```python
from build123d import *

# Parameters (mm, degrees)
SOCKETRIGHT_R                       = 16.7005
SOCKETRIGHT_DEPTH                   = 31.4325
SOCKETRIGHT_PITCH_ANGLE             = 90
SOCKETTOP_R                         = 16.7005
SOCKETTOP_DEPTH                     = 31.4325
SOCKETBOTTOM_R                      = 16.7005
SOCKETBOTTOM_DEPTH                  = 31.4325
SOCKETLEFT_R                        = 16.7005
SOCKETLEFT_DEPTH                    = 31.4325
SOCKETLEFT_PITCH_ANGLE              = 90
OBJ1_R           = 13.0683
OBJ1_DEPTH       = 108.2675
OBJ1_PITCH_ANGLE = 90
OBJ2             = 13.0683
OBJ3         = 108.2675
OBJ4_R           = 20.6375
OBJ4_DEPTH       = 98.425
OBJ4_PITCH_ANGLE = 90
OBJ5             = 20.6375
OBJ6         = 98.425


with BuildPart() as socketright:
    # SocketRight → SocketRight (new body)
    with BuildSketch(Plane.XY):
        Circle(SOCKETRIGHT_R)
    extrude(amount=SOCKETRIGHT_DEPTH)


with BuildPart() as socketright_1:
    # SocketRight pitch: moved
    add(socketright.part.rotate(Axis((0, 0, 0), (0, 1, 0)), SOCKETRIGHT_PITCH_ANGLE))


with BuildPart() as socketright_2:
    # SocketRight placement: moved
    add(socketright_1.part.moved(Location((20.6375, 0, 0))))


with BuildPart() as sockettop:
    # SocketTop → SocketTop (new body)
    with BuildSketch(Plane.XY.offset(20.6375)):
        Circle(SOCKETTOP_R)
    extrude(amount=SOCKETTOP_DEPTH)


with BuildPart() as socketbottom:
    # SocketBottom → SocketBottom (new body)
    with BuildSketch(Plane.XY.offset(-52.07)):
        Circle(SOCKETBOTTOM_R)
    extrude(amount=SOCKETBOTTOM_DEPTH)


with BuildPart() as sockets:
    # SocketLeft → SocketLeft (new body)
    with BuildSketch(Plane.XY):
        Circle(SOCKETLEFT_R)
    extrude(amount=SOCKETLEFT_DEPTH)


with BuildPart() as sockets_1:
    # SocketLeft pitch: moved
    add(sockets.part.rotate(Axis((0, 0, 0), (0, 1, 0)), SOCKETLEFT_PITCH_ANGLE))


with BuildPart() as sockets_2:
    # SocketLeft placement: moved
    add(sockets_1.part.moved(Location((-52.07, 0, 0))))

    # Sockets: union SocketRight, SocketTop, SocketBottom
    add(socketright_2.part)
    add(sockettop.part)
    add(socketbottom.part)


with BuildPart() as obj1:
    # obj1 → obj1 (new body)
    with BuildSketch(Plane.XY):
        Circle(OBJ1_R)
    extrude(amount=OBJ1_DEPTH)


with BuildPart() as obj1_1:
    # obj1 pitch: moved
    add(obj1.part.rotate(Axis((0, 0, 0), (0, 1, 0)), OBJ1_PITCH_ANGLE))


with BuildPart() as obj1_2:
    # obj1 placement: moved
    add(obj1_1.part.moved(Location((-54.13375, 0, 0))))


with BuildPart() as innercrossfusion:
    with BuildSketch(Plane.XY.offset(-54.13375)):
        Circle(OBJ2)
    extrude(amount=OBJ3)

    # InnerCrossFusion: union obj1
    add(obj1_2.part)


with BuildPart() as obj4:
    # obj4 → obj4 (new body)
    with BuildSketch(Plane.XY):
        Circle(OBJ4_R)
    extrude(amount=OBJ4_DEPTH)


with BuildPart() as obj4_1:
    # obj4 pitch: moved
    add(obj4.part.rotate(Axis((0, 0, 0), (0, 1, 0)), OBJ4_PITCH_ANGLE))


with BuildPart() as obj4_2:
    # obj4 placement: moved
    add(obj4_1.part.moved(Location((-49.2125, 0, 0))))


with BuildPart() as cross:
    with BuildSketch(Plane.XY.offset(-49.2125)):
        Circle(OBJ5)
    extrude(amount=OBJ6)

    # OuterCrossFusion: union obj4
    add(obj4_2.part)

    # Cut: cut InnerCrossFusion
    add(innercrossfusion.part, mode=Mode.SUBTRACT)

    # Cross: cut Sockets
    add(sockets_2.part, mode=Mode.SUBTRACT)


solid = cross.part
```
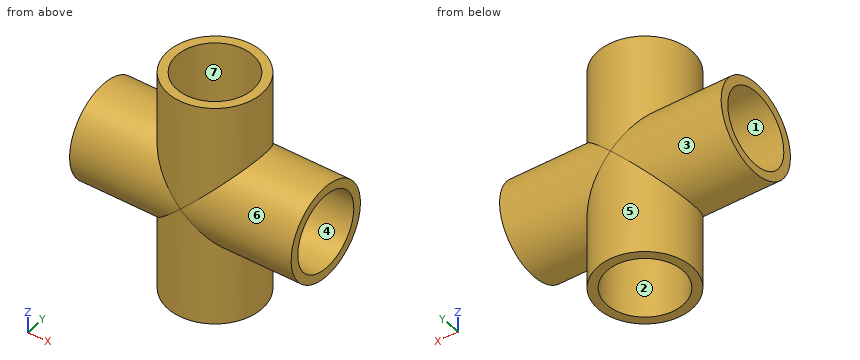
Geometry check sheet. Reference: the model listing, model coordinates, mm. Face numbers are marked on the shaded views. A direction names the side the tool comes from. Round coordinates to 2 decimals unless told otherwise and drop trailing zeros. Order: outer loops, then holes, each group sorted by start corner. A loop starts at its lowest first (then second) coordinate and runs counter-clockwise, first axis right, second up. Notation, with made-up numbers: (-2.75, 75.5) - (5.25, 75.5) arc R13 ccw to (5.25, 82.5) - close; hole circle Ø3 at (58.25, -10.75). An arc over 180 degrees is marked (long way). Use a Markdown table: item, result. Add a question column.
1) Section check A-A (z = 11.5). Record the cut outline in (x, y) (1 decimal), then the cut area to 3 significant figures.
2) Thickness scan on line 1 along Y through (x, z) = (-30.5, 0). Record the ranges inside material, lowest first.
3) Section check B-B (x = -15). Record the cut outline in (y, z) (1 decimal), then the cut area to 3 significant figures.
4) Section check D-D (z = -15). Record the cut outline in (x, y) (1 decimal).
5) Gauge pin test, flat ends, axial feed: P1, Ø20, axis at x = 0, y = 0, coming from the +Z side; P2, Ø12, axis at x = 1.5, z = -32, coming from the +Y side; P3, Ø16.5, axis at x = -3, y = -4.5, coming from the -Z side; P4, Ø6, axis at y = -15.5, z = -23.5, coming from the +X side. Record the tip position at first contact, or that the pin passes through.
6) Set-up check for the marked faces 5, 6 and 7: record each of +Z, -Z, +X, -X, +Y, -Y from which the full face is reachable in a straight line by a thin tool's end or side.
7) Mould release check, pull along Z, two halves, no side actions. Record for the marked faces 1, 2, 3 and 4: released by +Z, released by -Z, zero draft, split by the parting line, or undercut.
8) Section check C-C (y = 0). Count the separate pieces of the cut face and the enclosed holes in it, then the cut area to 3 significant figures.
Established:
| question | item | result |
|---|---|---|
| 1 | outline | (-49.2, -17.1) - (-11.5, -17.1) arc R20.6 ccw to (11.5, -17.1) - (49.2, -17.1) - (49.2, -12.1) - (20.6, -12.1) - (20.6, -6.2) - (11.5, -6.2) arc R13.1 cw to (-11.5, -6.2) - (-20.6, -6.2) - (-20.6, -12.1) - (-49.2, -12.1) - close; (-49.2, 12.1) - (-20.6, 12.1) - (-20.6, 6.2) - (-11.5, 6.2) arc R13.1 cw to (11.5, 6.2) - (20.6, 6.2) - (20.6, 12.1) - (49.2, 12.1) - (49.2, 17.1) - (11.5, 17.1) arc R20.6 ccw to (-11.5, 17.1) - (-49.2, 17.1) - close |
| 1 | area | 1,360 mm2 |
| 2 | line 1 | -20.64 to -16.7, 16.7 to 20.64 |
| 3 | outline | (-14.2, -49.2) - (-7.3, -49.2) - (-7.3, -20.6) - (7.3, -20.6) - (7.3, -49.2) - (14.2, -49.2) - (14.2, -15) arc R20.6 ccw to (14.2, 15) - (14.2, 49.2) - (7.3, 49.2) - (7.3, 20.6) - (-7.3, 20.6) - (-7.3, 49.2) - (-14.2, 49.2) - (-14.2, 15) arc R20.6 ccw to (-14.2, -15) - close; hole circle Ø26.1 at (0, 0) |
| 3 | area | 1,680 mm2 |
| 4 | outline | (-49.2, -14.2) - (-15, -14.2) arc R20.6 ccw to (15, -14.2) - (49.2, -14.2) - (49.2, -7.3) - (20.6, -7.3) - (20.6, 7.3) - (49.2, 7.3) - (49.2, 14.2) - (15, 14.2) arc R20.6 ccw to (-15, 14.2) - (-49.2, 14.2) - (-49.2, 7.3) - (-20.6, 7.3) - (-20.6, -7.3) - (-49.2, -7.3) - close; hole circle Ø26.1 at (0, 0) |
| 5 | P1 | through |
| 5 | P2 | y = 20.64 |
| 5 | P3 | z = -20.64 |
| 5 | P4 | x = 16.42 |
| 6 | face 5 | -Z |
| 6 | face 6 | +X |
| 6 | face 7 | +Z |
| 7 | face 1 | undercut |
| 7 | face 2 | zero draft |
| 7 | face 3 | split by the parting line |
| 7 | face 4 | undercut |
| 8 | separate pieces | 4 |
| 8 | enclosed holes | 0 |
| 8 | area | 1,130 mm2 |
